from build123d import *

# Parameters (mm, degrees)
F1_DEPTH = 12
F2_R     = 12.39
F3_DEPTH = 120


with BuildPart() as f1:
    # F0 (on Front) → F1 (new body)
    with BuildSketch(Plane.XZ):
        Polygon((-0.24929, 21.200885), (-18.48515, 10.384551), (-18.23586, -10.816334), (0.24929, -21.200885), (18.48515, -10.384551), (18.23586, 10.816334), align=None)
    extrude(amount=-F1_DEPTH)

    # F2 (on face) → F3 (join)
    with BuildSketch(Plane.XZ):
        Circle(F2_R)
    extrude(amount=F3_DEPTH)


solid = f1.part
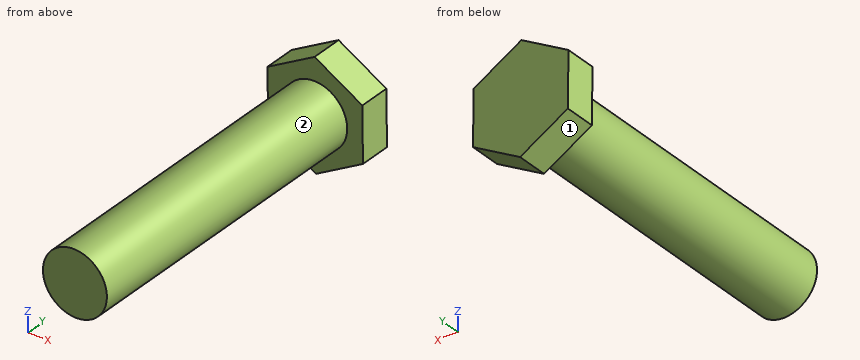
For this review, take the finished solid that the model builds, in its own axes (mm). Face numbers are marked on the shaded views. A direction names the side the tool comes from. Round coordinates to 2 decimals unless told otherwise and drop trailing zeros. Loops run counter-clockwise (first coordinate to the right, second up) from the corner with the lowest first, then second, coordinate; pieces in that order, holes last. Notation, with made-up numbers: (45, 8) - (98, 8) arc R15 ccw to (98, 25) - close; hole circle Ø7 at (59, 74). An arc over 180 degrees is marked (long way). Answer as CSV lines item,"result".
(1) Consider section B-B on z = 0. Give the boundary of the cut face in (x, y).
Checked values:
outline,"(-18.36, 0) - (-12.39, 0) - (-12.39, -120) - (12.39, -120) - (12.39, 0) - (18.36, 0) - (18.36, 12) - (-18.36, 12) - close"
(2) Consider section D-D on x = -15. Give the boundary of the cut face in (y, z), then the cut area to 3 significant figures.
Checked values:
outline,"(0, -12.63) - (12, -12.63) - (12, 12.45) - (0, 12.45) - close"
area,"301 mm2"
(3) Insertion check: P1, Ø4, axis at y = -98.5, z = 3.5, coming from the -X side; P2, Ø10, axis at x = 0.5, y = -98, coming from the -Z side; P3, Ø4, axis at y = -97.5, z = 5.5, coming from the +X side. Each pin has a flat end and moves straight along its axis. Give the tip position at first contact, or say it passes through.
Checked values:
P1,"stops at x = -12.3"
P2,"stops at z = -12.39"
P3,"stops at x = 11.89"
(4) Consider section C-C on y = -92. Give the boundary of the cut face in (x, z).
Checked values:
outline,"circle Ø24.78 at (0, 0)"
(5) Consider section A-A on x = 5.5. Give the boundary of the cut face in (y, z), then the cut area to 3 significant figures.
Checked values:
outline,"(-120, -11.1) - (0, -11.1) - (0, -18.09) - (12, -18.09) - (12, 17.97) - (0, 17.97) - (0, 11.1) - (-120, 11.1) - close"
area,"3,100 mm2"
(6) Tool access review of the marked faces 1 and 2: name each direction out of +Z, -Z, +X, -X, +Y, -Y from which nothing blocks a thin tool from reaching the whole face with its end or side.
Checked values:
face 1,"-Z, -X, +Y, -Y"
face 2,"-Y"
(7) Wall thickness on line 1 (Y direction, x = 4, z = 16); line 2 (X direction, y = -38, z = 6); line 3 (X direction, y = -9, z = -11.5): over which ranges is each line inside the solid? List them lowest first.
Checked values:
line 1,"y = 0 to 12"
line 2,"x = -10.84 to 10.84"
line 3,"x = -4.61 to 4.61"
